Geometry: final body of the model. Coordinates: model frame, mm. A direction names the side the tool comes from. Give positions to 0.01 mm unless a question says otherwise; leave off trailing zeros. Loops run counter-clockwise (first coordinate to the right, second up) from the corner with the lowest first, then second, coordinate; pieces in that order, holes last. Notation, with made-up numbers: (-14.75, 20.5) - (8.25, 20.5) arc R21 cw to (8.25, 45.5) - close; hole circle Ø11 at (86, 37). An arc over 180 degrees is marked (long way). Answer in a Markdown table with one row per item.
Autodesk Inventor part; units mm, degrees
ref_plane "YZ Plane" through (0, 0, 0) normal (1, 0, 0) x (0, 1, 0)
ref_plane "XZ Plane" through (0, 0, 0) normal (0, 1, 0) x (-1, 0, 0)
ref_plane "XY Plane" through (0, 0, 0) normal (0, 0, 1) x (1, 0, 0)
sketch "Sketch1" plane through (0, 0, 0) normal (1, 0, 0) x (0, 1, 0)
  line L0 (-1.299, -2.25) -> (-2.5981, 0)
  line L1 (-2.5981, 0) -> (-1.299, 2.25)
  line L2 (-1.299, 2.25) -> (1.299, 2.25)
  line L3 (1.299, 2.25) -> (2.5981, 0)
  line L4 (2.5981, 0) -> (1.299, -2.25)
  line L5 (1.299, -2.25) -> (-1.299, -2.25)
  line L6 (-2.829, -4.9) -> (-5.658, 0)
  line L7 (-5.658, 0) -> (-2.829, 4.9)
  line L8 (-2.829, 4.9) -> (2.829, 4.9)
  line L9 (2.829, 4.9) -> (5.658, 0)
  line L10 (5.658, 0) -> (2.829, -4.9)
  line L11 (2.829, -4.9) -> (-2.829, -4.9)
  point P0 (0, 0)
  point P1 (0, 0)
  point P2 (0, 0)
  dimension "d0" = 4.5
  dimension "d1" = 9.8
extrude "Extrusion1" add sketch "Sketch1" along normal blind 8
properties part number "Adaptador Acoplador" material "ABS Plastic"
Q1. Cut plane D-D (z = -3.75). Output: boundary loops of the cut face in (x, y).
Check values:
| item | result |
|---|---|
| outline | (0, -3.49) - (8, -3.49) - (8, 3.49) - (0, 3.49) - close |
Q2. Cut plane A-A (x = 2.5). Output: boundary loops of the cut face in (y, z).
Check values:
| item | result |
|---|---|
| outline | (-5.66, 0) - (-2.83, -4.9) - (2.83, -4.9) - (5.66, 0) - (2.83, 4.9) - (-2.83, 4.9) - close; hole (-2.6, 0) - (-1.3, -2.25) - (1.3, -2.25) - (2.6, 0) - (1.3, 2.25) - (-1.3, 2.25) - close |
Q3. Material intervals for line 1 along Z through (x, y) = (6.25, -1.25); line 2 along Y through (x, z) = (6.25, 1.25); line 3 along Z through (x, y) = (3.25, -1.5), sorted ascending.
Check values:
| item | result |
|---|---|
| line 1 | -4.9 to -2.25, 2.25 to 4.9 |
| line 2 | -4.94 to -1.88, 1.88 to 4.94 |
| line 3 | -4.9 to -1.9, 1.9 to 4.9 |
Q4. Cut plane C-C (z = -0.5). Output: boundary loops of the cut face in (x, y).
Check values:
| item | result |
|---|---|
| outline | (0, -5.37) - (8, -5.37) - (8, -2.31) - (0, -2.31) - close; (0, 2.31) - (8, 2.31) - (8, 5.37) - (0, 5.37) - close |
Q5. Draft query along Y for faces 3 (the flat face through (3.94, 4.26, -2.42)), 4 (the flat face through (3.94, -1.94, -1.14)), 5 (the flat face through (4, 0, -4.9)). Return one class per face: pulls with the +Y half, pulls with the -Y half, needs draft (parallel to the pull), parting line crosses it, or undercut.
Check values:
| item | result |
|---|---|
| face 3 | pulls with the +Y half |
| face 4 | undercut |
| face 5 | needs draft |
Q6. First-contact query: pin 1 (1.5 mm diameter, centred on x = 2.5, z = -4, fed in from +Y). Flat tip, straight axial feed; report the tip coordinate or a pass-through.
Check values:
| item | result |
|---|---|
| pin 1 | y = 3.78 |
Q7. Cut plane B-B (y = 0.25). Output: boundary loops of the cut face in (x, z).
Check values:
| item | result |
|---|---|
| outline | (0, -4.9) - (8, -4.9) - (8, -2.25) - (0, -2.25) - close; (0, 2.25) - (8, 2.25) - (8, 4.9) - (0, 4.9) - close |
Q8. Reachability of faces 1 (the flat face through (4, 0, -2.25)), 2 (the flat face through (3.944, 4.224, 2.484)) from +Z, -Z, +X, -X, +Y, -Y: full face, straight path, thin tool, end or side. Return the list, or none.
Check values:
| item | result |
|---|---|
| face 1 | +X, -X |
| face 2 | +Z, +X, -X, +Y |
